from build123d import *

# Parameters (mm, degrees)
BOSS_EXTRU_1_DEPTH = 10
ESQUISSE2_R        = 5
BOSS_EXTRU_2_DEPTH = 30
ESQUISSE3_R        = 5
BOSS_EXTRU_3_DEPTH = 30


with BuildPart() as part:
    # Esquisse1 → Boss.-Extru.1 (new body)
    with BuildSketch(Plane(origin=(0, 0, 0), x_dir=(1, 0, 0), z_dir=(0, 1, 0))):
        Polygon((0, 0), (189, 0), (189, 250), (0, 250), (0, 220), (-30, 220), (-30, 30), (0, 30), align=None)
    extrude(amount=BOSS_EXTRU_1_DEPTH)

    # Esquisse2 → Boss.-Extru.2 (add)
    with BuildSketch(Plane.XY.offset(-30)):
        with Locations((-25, 5)):
            Circle(ESQUISSE2_R)
    extrude(amount=BOSS_EXTRU_2_DEPTH)

    # Esquisse3 → Boss.-Extru.3 (add)
    with BuildSketch(Plane(origin=(0, 0, -220), x_dir=(-1, 0, 0), z_dir=(0, 0, -1))):
        with Locations((25, 5)):
            Circle(ESQUISSE3_R)
    extrude(amount=BOSS_EXTRU_3_DEPTH)


solid = part.part
Verification items for the finished model (mm, model axes). A direction names the side the tool comes from. Round coordinates to 2 decimals unless told otherwise and drop trailing zeros. Loops run counter-clockwise (first coordinate to the right, second up) from the corner with the lowest first, then second, coordinate; pieces in that order, holes last. Notation, with made-up numbers: (70.5, 66.25) - (122.5, 66.25) arc R16 cw to (122.5, 81.25) - close; hole circle Ø8 at (3.25, -13). An arc over 180 degrees is marked (long way). Answer in a Markdown table with one row per item. Add a question column.
Q1. Material ranges on line 1 (Z direction, x = -10, y = 8.25); line 2 (X direction, y = 8.5, z = -231.5), recorded low to high.
Q2. Gauge pin test, flat end, axial feed: pin 1 (3 mm diameter, centred on x = -8, y = 5.5, fed in from +Z). Record the tip position at first contact, or that the pin passes through.
Q3. Tool access check on faces 1 (the face through (-30, 5, -15)), 2 (the face through (-29, 1, -220)), 3 (the face through (0, 5, -15)), 4 (the face through (-20, 5, -235)), 5 (the face through (-29, 1, -30)). Record the directions out of +Z, -Z, +X, -X, +Y, -Y that give a thin tool (end or side, any length) a straight path to the whole face; none if there is none.
Q4. Section check A-A on z = -226.5. Enter the section's corners in (x, y).
Q5. Section check B-B on y = 1.5. Enter the section's corners in (x, z).
Found:
| question | item | result |
|---|---|---|
| 1 | line 1 | z = -220 to -30 |
| 1 | line 2 | x = -28.57 to -21.43, 0 to 189 |
| 2 | pin 1 | stops at z = -30 |
| 3 | face 1 | +Z |
| 3 | face 2 | -Z, -X, -Y |
| 3 | face 3 | +Z, +Y, -Y |
| 3 | face 4 | -Z |
| 3 | face 5 | +Z, -X, -Y |
| 4 | outline | circle Ø10 at (-25, 5); (0, 0) - (189, 0) - (189, 10) - (0, 10) - close |
| 5 | outline | (-30, -220) - (-28.57, -220) - (-28.57, -250) - (-21.43, -250) - (-21.43, -220) - (0, -220) - (0, -250) - (189, -250) - (189, 0) - (0, 0) - (0, -30) - (-21.43, -30) - (-21.43, 0) - (-28.57, 0) - (-28.57, -30) - (-30, -30) - close |
